For this review, use the dimensioned drawing (mm, ordinates from the lowest corner) and the shaded views. A direction names the side the tool comes from. Coordinates: 2 decimals unless noted, no trailing zeros. Loops run counter-clockwise (first coordinate to the right, second up) from the corner with the lowest first, then second, coordinate; pieces in that order, holes last. Notation, with made-up numbers: (24.25, 29) - (74.25, 29) arc R15 cw to (74.25, 38) - close; hole circle Ø5 at (8.5, 49). An arc over 180 degrees is marked (long way). Answer in a Markdown table with one row per item. Add a question column.
(1) The part is to be moulded in two halves that separate along Z. For the marked faces 1, 2 and 3, say which applies: released by +Z, released by -Z, zero draft, split by the parting line, or undercut.
(2) For the marked faces 4 and 5, list the 3-axis set-ups (+Z, -Z, +X, -X, +Y, -Y) from which the entire face can be reached by the end or side of a thin tool; tool diameter is ignored.
(3) We need section A-A, the plane z = 21. Give the number of separate pieces and of enclosed holes in the cut face.
(4) To check wall thickness, follow L1, parallel to X at y = 2.75, z = 13.5 (1 decimal); L2, parallel to Z at x = 8.5, y = 1; L3, parallel to X at y = 3.25, z = 26.5 (1 decimal). State the ranges of each line that lie inside material, in increasing order. Write a range as [from, to].
(5) We need section B-B, the plane y = 4.75. Write out the cut boundary in (x, z) (1 decimal).
(6) Clearance check with a flat-ended pin moving along its axis: pin 1 (3 mm diameter, centred on y = 3.5, z = 18.5, fed in from -X). State where the tip first meets the part, or that it passes through.
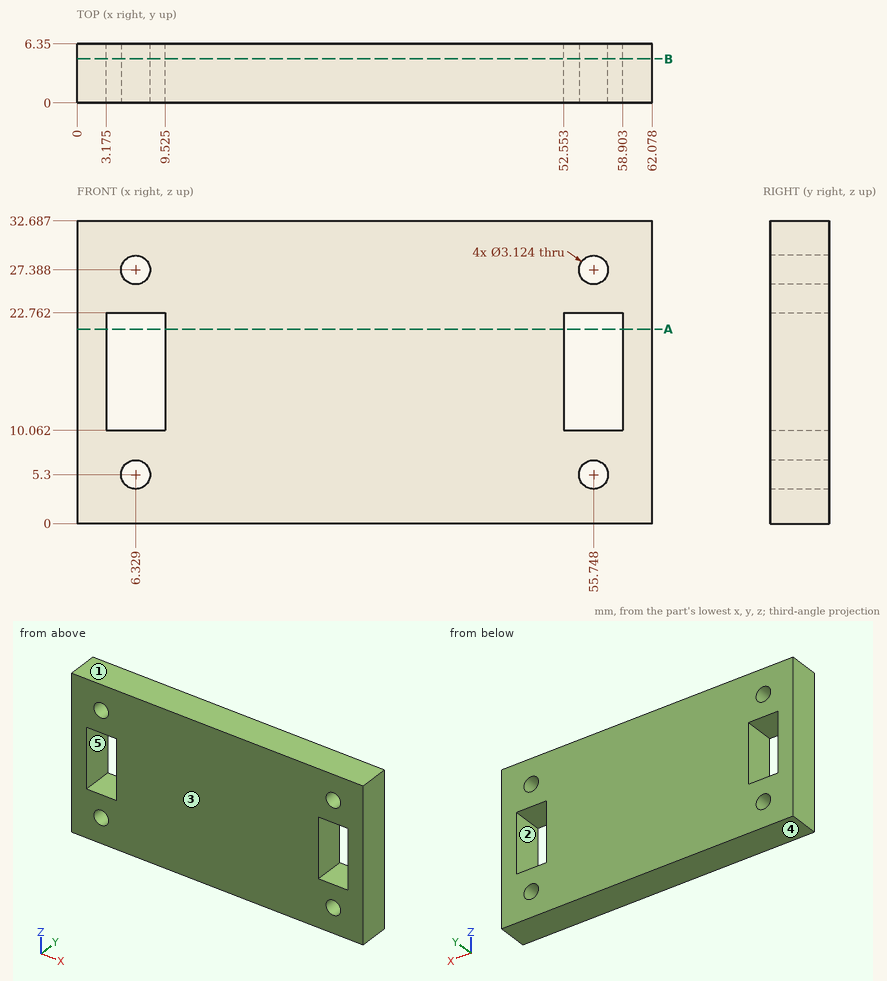
Responses:
| question | item | result |
|---|---|---|
| 1 | face 1 | released by +Z |
| 1 | face 2 | undercut |
| 1 | face 3 | zero draft |
| 2 | face 4 | -Z, +X, -X, +Y, -Y |
| 2 | face 5 | +Y, -Y |
| 3 | separate pieces | 3 |
| 3 | enclosed holes | 0 |
| 4 | L1 | x = [0, 3.2], [9.5, 52.6], [58.9, 62.1] |
| 4 | L2 | z = [0, 10.06], [22.76, 32.69] |
| 4 | L3 | x = [0, 5], [7.6, 54.5], [57, 62.1] |
| 5 | outline | (0, 0) - (62.1, 0) - (62.1, 32.7) - (0, 32.7) - close; hole (3.2, 10.1) - (9.5, 10.1) - (9.5, 22.8) - (3.2, 22.8) - close; hole circle Ø3.1 at (6.3, 5.3); hole circle Ø3.1 at (6.3, 27.4); hole (52.6, 10.1) - (58.9, 10.1) - (58.9, 22.8) - (52.6, 22.8) - close; hole circle Ø3.1 at (55.7, 5.3); hole circle Ø3.1 at (55.7, 27.4) |
| 6 | pin 1 | stops at x = 0 |
